Read the model definition and answer for the solid it produces. Units are mm, in the model's axes. A direction names the side the tool comes from. Coordinates: 2 decimals unless noted, no trailing zeros. Loops run counter-clockwise (first coordinate to the right, second up) from the corner with the lowest first, then second, coordinate; pieces in that order, holes last.
from build123d import *

# Parameters (mm, degrees)
PACK_SARJOR_L_KILAVUZ_2_1_START = 1040
PACK_SARJOR_L_KILAVUZ_2_1_DEPTH = 840


with BuildPart() as part:
    # Sketch1 → PACK_sarjor_L_kilavuz_2_1 (new body)
    with BuildSketch(Plane(origin=(0, 0, 0), x_dir=(1, 0, 0), z_dir=(0, 1, 0)).offset(PACK_SARJOR_L_KILAVUZ_2_1_START)):
        Polygon((560, 800), (550, 800), (550, 798), (558, 798), (558, 20), (560, 20), align=None)
    extrude(amount=PACK_SARJOR_L_KILAVUZ_2_1_DEPTH)


solid = part.part
Q1. Straight lines are drawn through the part: probe 1 along X at (y, z) = (1187, -310.5); probe 2 along Z at (x, y) = (556.25, 1670). For each, find the intervals that lie inside material, in ascending order.
Findings below:
probe 1: x = 558 to 560
probe 2: z = -800 to -798
Q2. A cutting plane is placed at A-A (y = 1460). Give the vertices of the cut face in (x, z), then the cut area to 3 significant figures.
Findings below:
outline: (550, -800) - (560, -800) - (560, -20) - (558, -20) - (558, -798) - (550, -798) - close
area: 1,580 mm2
Q3. A cutting plane is placed at B-B (z = -609.5). Give the vertices of the cut face in (x, y).
Findings below:
outline: (558, 1040) - (560, 1040) - (560, 1880) - (558, 1880) - close
Q4. Flat-ended cylindrical pins translate along their axes: pin 1 Ø3 at (x, y) = (551.5, 1142.5) entering from +Z; pin 2 Ø4 at (x, z) = (555, -385) entering from +Y. Find the tip coordinate at first contact, or state that the pin passes through.
Findings below:
pin 1: stops at z = -798
pin 2: passes through
Q5. A cutting plane is placed at C-C (x = 555). Give the vertices of the cut face in (y, z).
Findings below:
outline: (1040, -800) - (1880, -800) - (1880, -798) - (1040, -798) - close
Q6. Which of the six approach directions +Z, -Z, +X, -X, +Y, -Y give full straight-line access (tool end or side, diameter ignored) to faces 1 (the face through (558, 1454, -414)), 2 (the face through (560, 1454, -405))?
Findings below:
face 1: +Z, -X, +Y, -Y
face 2: +Z, -Z, +X, +Y, -Y
